CAD build for the part. Positions are in the model's coordinates, mm. A direction names the side the tool comes from. Give positions to 0.01 mm unless a question says otherwise; leave off trailing zeros. Write each loop counter-clockwise with the first axis right and the second up, starting at its lowest first coordinate (ties: lowest second). Pieces come first, ordered by that corner, then holes. Notation, with made-up numbers: (70.25, -22) - (98.25, -22) arc R5 ccw to (98.25, -17) - close; hole circle Ø2 at (-31, -10). An arc over 180 degrees is marked (long way). Answer as a JSON object with one key per item and string values.
Autodesk Inventor part; units mm, degrees
ref_plane "Work Plane1" through (1.525, 0, 0) normal (0, 0, 1) x (1, 0, 0)
ref_plane "YZ Plane" through (0, 0, 0) normal (1, 0, 0) x (0, 1, 0)
ref_plane "XZ Plane" through (0, 0, 0) normal (0, 1, 0) x (-1, 0, 0)
sketch "Sketch1" plane through (0, 0, 0) normal (0, 0, 1) x (1, 0, 0)
  line L0 (0, 4) -> (85, 4)
  line L1 (85, 4) -> (85, 0)
  line L2 (85, 0) -> (0, 0)
  line L3 (-14, 0) -> (84, 0)
  line L4 (0, -0.8) -> (0, 4.8)
  line L5 (0, 4) -> (0, 0)
  dimension "d2" = 8
  dimension "d59" = 85
revolve "Body" add sketch "Sketch1" angle 360 about axis through (85, 0, 0) along (-1, 0, 0)
sketch "Sketch2" plane through (0, 0, 0) normal (-1, 0, 0) x (0, 0, 1)
  line L0 (0, 7.5056) -> (6.5, 3.7528)
  line L1 (6.5, 3.7528) -> (6.5, -3.7528)
  line L2 (6.5, -3.7528) -> (0, -7.5056)
  line L3 (0, -7.5056) -> (-6.5, -3.7528)
  line L4 (-6.5, -3.7528) -> (-6.5, 3.7528)
  line L5 (-6.5, 3.7528) -> (0, 7.5056)
  line L6 (-9.1, 0) -> (9.1, 0)
  line L7 (0, 10.5078) -> (0, -10.5078)
  point P0 (0, 0)
  point P1 (0, 0)
  dimension "d11" = 13
extrude "Head" add sketch "Sketch2" along normal blind 5.68
sketch "Sketch4" plane through (0, 0, 0) normal (0, 0, 1) x (1, 0, 0)
  line L0 (-4.9294, 7.8) -> (-5.68, 6.5)
  line L1 (-1.1, 0) -> (-0.234, 0)
  line L2 (-6.7692, 0) -> (0.8552, 0)
  line L3 (-5.68, 7.8) -> (-4.9294, 7.8)
  line L4 (-5.68, 6.5) -> (-5.68, 7.8)
  line L5 (0, 9.36) -> (0, -1.56)
  dimension "d65" = 13
  dimension "d67" = 30
  dimension "d68" = 15.6
  dimension "d69" = 5.68
revolve "Chamfer1" cut sketch "Sketch4" angle 360 about axis through (-1.1, 0, 0) along (1, 0, 0)
thread "Thread"
chamfer "Chamfer2" distance 0.7668 distance2 0.7669 1 edges at (85, -4, 0) measured on face at (85, -0.4728, -1.2467)
fillet "Fillet" radius 0.1 1 edges at (0, -4, 0)
ref_plane "Work Plane1" through (1.525, 0, 0) normal (0, 0, 1) x (1, 0, 0)
equation "\"d2\" = GD"
equation "\"d59\" = NLG"
equation "\"d11\" = SW"
equation "\"d3\" = KOH"
equation "\"d15\" = GEL"
equation "\"d6\" = -0.5 * SPD + 0.5 * GD"
equation "\"d71\" = RR"
equation "\"d65\" = SW"
equation "\"d67\" = ANG1"
equation "\"d68\" = 1.2 * SW"
equation "\"d69\" = KOH"
equation "\"NLG\" = 85"
equation "\"GD\" = NND"
equation "\"BDM\" = NND"
equation "\"KOH\" = 5.68"
equation "\"GEL\" = 22"
equation "\"SW\" = 13"
equation "\"SW0\" = SW"
equation "\"SPD\" = NND - 1.2269 * PTC"
equation "\"SD2\" = NND"
equation "\"SD\" = 0"
equation "\"ANG1\" = 30deg"
equation "\"GAL\" = 0.61345 * PTC"
equation "\"GUL\" = 0.61345 * PTC"
equation "\"RR\" = 0.1"
equation "\"RR1\" = 0.4"
equation "\"GD1\" = THREADDIA - 1.2269 * PTC"
equation "\"THREADDIA\" = 8"
equation "\"TOA\" = 30deg"
equation "\"PTC\" = 1.25"
equation "\"KOH1\" = 3.7"
equation "\"NND\" = 8"
equation "\"E0\" = 1.155 * SW"
properties part number "M8x85" material "Steel, Mild"
(1) 3-axis set-ups, long thin cutter, end or side, ignore diameter. For faces 1 (the face through (-3, 0, 6.5)), 2 (the face through (0, -3.2, 2.8)): which of +Z, -Z, +X, -X, +Y, -Y reach the whole face in a straight line?
Answer key:
{"face 1": "+Z, +X, -X, +Y, -Y", "face 2": "+X"}
(2) Saw through at A-A, the plane x = 37.5. Give the cut face in (y, z), and give its area (3 significant figures).
Answer key:
{"outline": "circle Ø8 at (0, 0)", "area": "50.3 mm²"}
(3) Flat gauge pins, fed straight in: P1, Ø6, axis at x = 60, y = 0, coming from the +Z side; P2, Ø1, axis at x = 11, y = 3.5, coming from the +Z side; P3, Ø6, axis at y = 6, z = 2, coming from the +X side. Where does each tip first touch, or does it go through?
Answer key:
{"P1": "stops at z = 4", "P2": "stops at z = 2.65", "P3": "stops at x = 84.91"}
(4) Probe L1, parallel to X at y = -4.25, z = 0.25; L2, parallel to Y at x = 73, z = -0.25; L3, parallel to Z at x = 69, y = 3. List the from-to ranges inside material, lowest first. Write a range as [from, to].
Answer key:
{"L1": "x = [-5.68, 0]", "L2": "y = [-3.99, 3.99]", "L3": "z = [-2.65, 2.65]"}
